from build123d import *

# Parameters (mm, degrees)
EXTRUDE_2338_DEPTH = 2


with BuildPart() as part:
    # Sketch 227 → Повернуть1 (revolve)
    with BuildSketch(Plane.XY, mode=Mode.PRIVATE) as revolve_1_sk:
        with BuildLine():
            Line((6, 10), (1, 10))
            Line((1, 10), (1, 0))
            Line((1, 0), (2, 0))
            Line((2, 0), (2, 5.25))
            Line((2, 5.25), (4.5, 5.25))
            Line((4.5, 5.25), (4.5, 0))
            Line((4.5, 0), (11.2, 0))
            Line((11.2, 0), (11.2, 4.8))
            ThreePointArc((11.2, 4.8), (10.2627417, 7.0627417), (8, 8))
            ThreePointArc((8, 8), (7.414213562, 9.414213562), (6, 10))
        make_face()
    revolve(revolve_1_sk.sketch.rotate(Axis((0, 0, 0), (1, 0, 0)), 90), axis=Axis((0, 0, 0), (1, 0, 0)))

    # Sketch 1321 → Extrude 2338 (add, symmetric)
    with BuildSketch(Plane.XY):
        with BuildLine():
            ThreePointArc((11.2, 4.4), (29.338267199, 10.995701086), (45.2, 0))
            Line((45.2, 0), (11.2, 0))
            Line((11.2, 0), (11.2, 4.4))
        make_face()
        with BuildLine():
            Line((31.263463773, 0), (11.2, 0))
            Line((11.2, 0), (11.2, -3.914978255))
            ThreePointArc((11.2, -3.914978255), (22.080678837, -6.30816882), (31.263463773, 0))
        make_face()
        Polygon((38.912013935, 0), (35.248695767, 0), (35.248695767, -11.07), (38.912013935, -4.32), align=None)
        Polygon((35.248695767, 0), (31.263463773, 0), (32.498964702, -1.197255299), (32.498964702, -9.797255299), (35.248695767, -11.07), align=None)
        Polygon((42.083014277, -1.2), (42.083014277, 0), (40.307542508, 0), (40.307542508, -6.49), align=None)
        Polygon((40.307542508, 0), (38.912013935, 0), (38.912013935, -4.32), (40.307542508, -6.49), align=None)
        Polygon((42.083014277, -1.2), (45.2, 0), (42.083014277, 0), align=None)
    extrude(amount=EXTRUDE_2338_DEPTH, both=True)


solid = part.part
Design review of the part built by this model. Coordinates are the model's own, in mm. A direction names the side the tool comes from. Round coordinates to 2 decimals unless told otherwise and drop trailing zeros. Order: outer loops, then holes, each group sorted by start corner. A loop starts at its lowest first (then second) coordinate and runs counter-clockwise, first axis right, second up.
1) Consider section B-B (x = 29). State the section outline as (y, z) points, plus the area to 3 significant figures.
The answers:
outline: (-2.76, -2) - (11.04, -2) - (11.04, 2) - (-2.76, 2) - close
area: 55.2 mm2
2) Clearance check with flat-ended pins moving along their axes: pin 1 Ø8 at (x, y) = (36, -4) entering from -Z; pin 2 Ø12 at (x, y) = (12, 5) entering from +Z; pin 3 Ø6 at (x, y) = (15, -0.5) entering from +Z; pin 4 Ø1.5 at (x, y) = (12, 7) entering from +Z. State where each tip first meets the part, or that it passes through.
The answers:
pin 1: stops at z = -2
pin 2: stops at z = 9.63
pin 3: stops at z = 2
pin 4: passes through
3) Draft analysis for pull direction Z (two halves, no side actions). For faces 4 (the flat face through (41.183, -3.882, 0.028)), 5 (the flat face through (2, 0, 0)), 6 (the flat face through (28, 3, -2)), 7 (the flat face through (4.5, 0, 0)), state which applies: released by +Z, released by -Z, zero draft, split by the parting line, or undercut.
The answers:
face 4: zero draft
face 5: undercut
face 6: released by -Z
face 7: undercut
4) Consider section D-D (x = 7). State the section outline as (y, z) points.
The answers:
outline: circle Ø19.46 at (0, 0)
5) Consider section C-C (x = 36.5). State the section outline as (y, z) points, plus the area to 3 significant figures.
The answers:
outline: (-8.76, -2) - (8.71, -2) - (8.71, 2) - (-8.76, 2) - close
area: 69.9 mm2
6) Machinability: for faces 1 (the flat face through (32.499, -5, 0)), 2 (the cylindrical face through (3.3, -1.6, 5)), 3 (the flat face through (28, 3, 2)), which of the approach directions +Z, -Z, +X, -X, +Y, -Y give a long, thin tool a straight path to every point of the face, cutting with its end or side? Answer none if there is none.
The answers:
face 1: +Z, -Z, -Y
face 2: none
face 3: +Z, +X, +Y, -Y
7) For L1, parallel to Y at x = 3.15, z = 0; L2, parallel to Z at x = 12.5, y = -1; L3, parallel to X at y = -0.5, z = -2.5, list the stretches that pass through material, from the lowest coordinate up.
The answers:
L1: y = -10 to -5.25, 5.25 to 10
L2: z = -2 to 2
L3: x = 1 to 2, 4.5 to 11.2
8) Consider section A-A (z = 0). State the section outline as (x, y) points.
The answers:
outline: (1, -10) - (6, -10) arc R2 ccw to (8, -8) arc R3.2 ccw to (11.2, -4.8) - (11.2, -3.91) arc R14 ccw to (31.26, 0) - (32.5, -1.2) - (32.5, -9.8) - (35.25, -11.07) - (38.91, -4.32) - (40.31, -6.49) - (42.08, -1.2) - (45.2, 0) arc R21 ccw to (11.2, 4.4) - (11.2, 4.8) arc R3.2 ccw to (8, 8) arc R2 ccw to (6, 10) - (1, 10) - close; hole (2, -5.25) - (4.5, -5.25) - (4.5, 5.25) - (2, 5.25) - close
